```python
from build123d import *

# Parameters (mm, degrees)
SKETCH4_R           = 50
SKETCH4_R_2         = 45
BOSS_EXTRUDE2_DEPTH = 2.5
SKETCH6_R           = 22.25
SKETCH6_R_2         = 10
BOSS_EXTRUDE3_DEPTH = 2.5
BOSS_EXTRUDE4_DEPTH = 2.5
CIRPATTERN1_COUNT   = 4
CUT_EXTRUDE2_DEPTH  = 20
SKETCH19_R          = 1.25
CUT_EXTRUDE3_DEPTH  = 2.5
CIRPATTERN2_COUNT   = 4
SKETCH20_R          = 50
SKETCH20_R_2        = 45
BOSS_EXTRUDE5_DEPTH = 11


with BuildPart() as part:
    # Sketch4 → Boss-Extrude2 (new body, symmetric)
    with BuildSketch(Plane.XY):
        Circle(SKETCH4_R)
        Circle(SKETCH4_R_2, mode=Mode.SUBTRACT)
    extrude(amount=BOSS_EXTRUDE2_DEPTH, both=True)



with BuildPart() as body_2:
    # Sketch6 → Boss-Extrude3 (new body, symmetric)
    with BuildSketch(Plane.XY):
        Circle(SKETCH6_R)
        Circle(SKETCH6_R_2, mode=Mode.SUBTRACT)
    extrude(amount=BOSS_EXTRUDE3_DEPTH, both=True)


with BuildPart() as part_1:
    add(part.part)

    add(body_2.part)  # Boss-Extrude4 merges body 2
    # Sketch7 → Boss-Extrude4 (add, symmetric)
    with BuildSketch(Plane.XY):
        with BuildLine():
            Line((1.5, 22.173723668), (1.5, 44.974993052))
            ThreePointArc((1.5, 44.974993052), (0, 45), (-1.5, 44.974993052))
            Line((-1.5, 44.974993052), (-1.5, 22.173723668))
            ThreePointArc((-1.5, 22.173723668), (0, 22.224401484), (1.5, 22.173723668))
        make_face()
    boss_extrude4 = extrude(amount=BOSS_EXTRUDE4_DEPTH, both=True)

    # CirPattern1: Boss-Extrude4 ×4 about axis
    cirpattern1_axis = Axis((0, 0, 0), (0, 0, 1))
    for i in range(1, CIRPATTERN1_COUNT):
        add(boss_extrude4.rotate(cirpattern1_axis, i * 360 / CIRPATTERN1_COUNT))

    # Sketch16 → Revolve5 (revolve)
    with BuildSketch(Plane(origin=(0, 0, 0), x_dir=(0, 0, -1), z_dir=(1, 0, 0))):
        with BuildLine():
            Line((2.5, 22.5), (2.5, 20))
            Line((2.5, 20), (8.319227557, 20))
            add(Edge.make_bspline(
                [(8.319227557, 20), (11.123254562, 19.6727407), (15.973153481, 19.619040378), (22.945159124, 18.263658856), (29.398925624, 16.810806242), (36.513582053, 14.385022759), (43.601684551, 11.54818751), (48.61668349, 9.827339582), (50.700170198, 8.605167266)],
                knots=[0, 0, 0, 0, 0.1918853, 0.327499488, 0.481339331, 0.640782173, 0.837003533, 1, 1, 1, 1], degree=3))
            add(Edge.make_bspline(
                [(50.700170198, 8.605167266), (51.227102493, 8.224080677), (51.754034788, 7.842994089)],
                knots=[0, 0, 0, 1, 1, 1], degree=2))
            Line((51.754034788, 7.842994089), (52.5, 7.303499091))
            Line((52.5, 7.303499091), (52.5, 10.388790167))
            add(Edge.make_bspline(
                [(52.068285629, 10.701013498), (52.122249925, 10.661985582), (52.284142815, 10.544901832), (52.446035704, 10.427818083), (52.5, 10.388790167)],
                knots=[-0.091980981, -0.091980981, -0.091980981, 0.010431221, 0.215255624, 0.317667825, 0.317667825, 0.317667825], degree=2))
            add(Edge.make_bspline(
                [(8.464622197, 22.5), (9.346604646, 22.397063417), (11.091341923, 22.245478983), (13.864723915, 22.08493702), (16.750982068, 21.863282745), (19.67100668, 21.437998985), (22.472128979, 20.890581106), (25.220298474, 20.307886272), (27.995926722, 19.661513734), (31.709227942, 18.654015601), (35.320256891, 17.428854793), (38.839343196, 16.113628139), (41.44099355, 15.113187926), (44.015827232, 14.123528369), (46.587421441, 13.193671921), (48.868261591, 12.319589328), (50.476081329, 11.570913159), (51.283275743, 11.147887794), (51.680089744, 10.926618218), (51.915375523, 10.790958684), (52.015905313, 10.731739767), (52.068285629, 10.701013498)],
                knots=[-0.003294191, -0.003294191, -0.003294191, -0.003294191, 0.059579874, 0.122453939, 0.185328004, 0.248202069, 0.311076134, 0.373950199, 0.436824265, 0.49969833, 0.62544646, 0.688320525, 0.75119459, 0.814068655, 0.87694272, 0.939816785, 0.971253818, 0.986972334, 0.994831592, 0.998761221, 1.00269085, 1.00269085, 1.00269085, 1.00269085], degree=3))
            Line((8.464622197, 22.5), (7.5, 22.5))
            Line((7.5, 22.5), (5, 22.5))
            Line((5, 22.5), (2.5, 22.5))
        make_face()
    revolve(axis=Axis((0, 0, -2.5), (0, 0, -1)))

    # Sketch17 → Cut-Extrude2 (cut)
    with BuildSketch(Plane.XY.offset(2.5)):
        with BuildLine():
            ThreePointArc((12.992330947, 11.923401399), (9.06375587, 16.758610598), (2.86682458, 17.399697733))
            ThreePointArc((2.86682458, 17.399697733), (0.852954159, 13.676112204), (4.576539687, 11.662241783))
            ThreePointArc((4.576539687, 11.662241783), (6.215713007, 11.492665443), (7.254874997, 10.213686293))
            ThreePointArc((7.254874997, 10.213686293), (10.978460525, 8.199815871), (12.992330947, 11.923401399))
        make_face()
        with BuildLine():
            ThreePointArc((11.923401399, -12.992330947), (16.758610598, -9.06375587), (17.399697733, -2.86682458))
            ThreePointArc((17.399697733, -2.86682458), (13.676112204, -0.852954159), (11.662241783, -4.576539687))
            ThreePointArc((11.662241783, -4.576539687), (11.492665443, -6.215713007), (10.213686293, -7.254874997))
            ThreePointArc((10.213686293, -7.254874997), (8.199815871, -10.978460525), (11.923401399, -12.992330947))
        make_face()
        with BuildLine():
            ThreePointArc((-12.992330947, -11.923401399), (-9.06375587, -16.758610598), (-2.86682458, -17.399697733))
            ThreePointArc((-2.86682458, -17.399697733), (-0.852954159, -13.676112204), (-4.576539687, -11.662241783))
            ThreePointArc((-4.576539687, -11.662241783), (-6.215713007, -11.492665443), (-7.254874997, -10.213686293))
            ThreePointArc((-7.254874997, -10.213686293), (-10.978460525, -8.199815871), (-12.992330947, -11.923401399))
        make_face()
        with BuildLine():
            ThreePointArc((-11.923401399, 12.992330947), (-16.758610598, 9.06375587), (-17.399697733, 2.86682458))
            ThreePointArc((-17.399697733, 2.86682458), (-13.676112204, 0.852954159), (-11.662241783, 4.576539687))
            ThreePointArc((-11.662241783, 4.576539687), (-11.492665443, 6.215713007), (-10.213686293, 7.254874997))
            ThreePointArc((-10.213686293, 7.254874997), (-8.199815871, 10.978460525), (-11.923401399, 12.992330947))
        make_face()
    extrude(amount=-CUT_EXTRUDE2_DEPTH, mode=Mode.SUBTRACT)

    # Sketch19 → Cut-Extrude3 (cut, symmetric)
    with BuildSketch(Plane(origin=(0, 47.5, 0), x_dir=(1, 0, 0), z_dir=(0, 1, 0))):
        Circle(SKETCH19_R)
    cut_extrude3 = extrude(amount=CUT_EXTRUDE3_DEPTH, both=True, mode=Mode.SUBTRACT)

    # CirPattern2: Cut-Extrude3 ×4 about axis
    cirpattern2_axis = Axis((0, 0, 0), (0, 0, 1))
    for i in range(1, CIRPATTERN2_COUNT):
        add(cut_extrude3.rotate(cirpattern2_axis, i * 360 / CIRPATTERN2_COUNT), mode=Mode.SUBTRACT)

    # Sketch20 → Boss-Extrude5 (add)
    with BuildSketch(Plane.XY.offset(2.5)):
        Circle(SKETCH20_R)
        Circle(SKETCH20_R_2, mode=Mode.SUBTRACT)
    extrude(amount=BOSS_EXTRUDE5_DEPTH)


solid = part_1.part
```
Model file for the job. Use its own axes, mm. A direction names the side the tool comes from. Coordinates: 2 decimals unless noted, no trailing zeros. Order: outer loops, then holes, each group sorted by start corner. A loop starts at its lowest first (then second) coordinate and runs counter-clockwise, first axis right, second up. Notation, with made-up numbers: (-7, 9.25) - (12, 9.25) arc R22 cw to (12, 25.25) - close; hole circle Ø9 at (36, 21.25). An arc over 180 degrees is marked (long way). Return JSON: item names as keys, results as strings. Group by question number.
1) Mould opens along Y. For faces 4 (the flat face through (-1.5, 34, 0)), 5 (the flat face through (0, -45, 0)), 6 (the flat face through (26, 0, -2.5)), 7 (the cylindrical face through (-15.574, 15.89, 0.035)) say: released by +Y, released by -Y, zero draft, split by the parting line, or undercut.
2) Tool access for faces 1 (the flat face through (2.5, 7.1, -52.5)), 2 (the cylindrical face through (-13.739, 0.835, 0.035)), 3 (the flat face through (9, 5, -2.5)): list every direction of +Z, -Z, +X, -X, +Y, -Y with a clear straight run to the whole face (end or side of a thin tool).
3) Flat gauge pins, fed straight in: P1, Ø5.5, axis at x = -34.5, z = -1, coming from the -Y side; P2, Ø18, axis at x = 0, y = 0, coming from the +Z side; P3, Ø1.5, axis at x = 29.5, z = 0, coming from the -Y side. Where does each tip first touch, or does it go through?
4) Saw through at C-C, the plane z = -5. Write the cut outline in (x, y).
5) Saw through at B-B, the plane x = 37.5. Write the cut outline in (y, z).
6) Saw through at A-A, the plane y = 29. Write the cut outline in (x, z).
7) Probe line 1 (Y direction, x = 0, z = 0); line 2 (Z direction, x = 47, y = 0); line 3 (X direction, y = 0, z = -4). List the from-to ranges inside material, lowest first. Write a range as from..to.
Values found:
{
 "1": {"face 4": "undercut", "face 5": "released by -Y", "face 6": "zero draft", "face 7": "undercut"},
 "2": {"face 1": "-Z, +X, -X, +Y, -Y", "face 2": "+Z", "face 3": "none"},
 "3": {"P1": "stops at y = -38.63", "P2": "stops at z = -49.99", "P3": "stops at y = -40.91"},
 "4": {"outline": "circle Ø45 at (0, 0); hole circle Ø40 at (0, 0)"},
 "5": {"outline": "(-33.07, -2.5) - (-24.87, -2.5) - (-24.87, 13.5) - (-33.07, 13.5) - close; (-1.5, -2.5) - (1.5, -2.5) - (1.5, 2.5) - (-1.5, 2.5) - close; (24.87, -2.5) - (33.07, -2.5) - (33.07, 13.5) - (24.87, 13.5) - close"},
 "6": {"outline": "(-40.73, -2.5) - (-34.41, -2.5) - (-34.41, 13.5) - (-40.73, 13.5) - close; (-1.5, -2.5) - (1.5, -2.5) - (1.5, 2.5) - (-1.5, 2.5) - close; (34.41, -2.5) - (40.73, -2.5) - (40.73, 13.5) - (34.41, 13.5) - close"},
 "7": {"line 1": "y = -45..-10, 10..45", "line 2": "z = -2.5..-1.25, 1.25..13.5", "line 3": "x = -22.5..-20, 20..22.5"}
}
